Can you work these out from the drawing? Everything is in mm from the part's minimum corner. Round coordinates to 2 decimals unless told otherwise and drop trailing zeros. Order: outer loops, then holes, each group sorted by start corner. A loop starts at its lowest first (then second) coordinate and runs counter-clockwise, first axis right, second up. Notation, with made-up numbers: M 30.5,18.25 L 43.5,18.25 A33 ccw 43.5,56.25 Z; hole C -38,24.25 d11. An arc over 180 degrees is marked long. Write item = value, one per line. Start each with the question number.
Item 1: Please list where these lines run through material, in increasing order: L1, parallel to X at y = 10.75, z = 329.5; L2, parallel to Y at x = 69, z = 673.5; L3, parallel to X at y = 1.75, z = 308.5.
Item 2: I want a section at B-B, the plane y = 13.75. List the corners of the cut face in (x, z) for me, plus the area to 3 significant figures.
Item 3: I'm going to push flat-ended pins straight in: P1, Ø3, axis at y = 9.5, z = 846.5, coming from the +X side; P2, Ø1, axis at x = 14.5, y = 8.5, coming from the -Z side; P3, Ø2, axis at y = 15, z = 793.5, coming from the +X side; P4, Ø1.5, axis at y = 15, z = 720.5, coming from the +X side. Where does each tip first touch, or does it pass through?
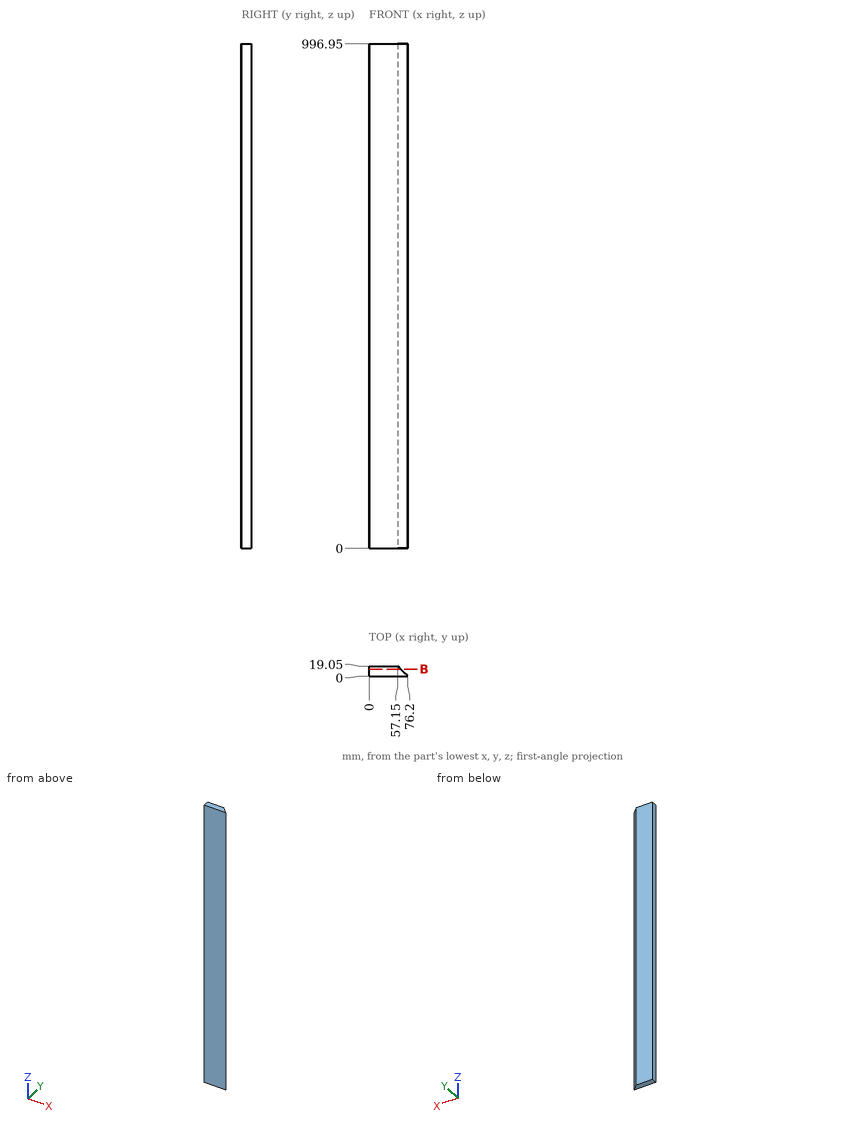
Filled in:
q1.L1 = 0 to 65.45
q1.L2 = 0 to 7.2
q1.L3 = 0 to 74.45
q2.outline = M 0,0 L 62.45,0 L 62.45,996.95 L 0,996.95 Z
q2.area = 62,300 mm^2
q3.P1 = 68.2
q3.P2 = 0
q3.P3 = 62.2
q3.P4 = 61.95
